from build123d import *

# Parameters (mm, degrees)
SKETCH1_R           = 17.5
BOSS_EXTRUDE1_DEPTH = 50
BOSS_EXTRUDE2_START = -50
SKETCH2_R           = 27.5
BOSS_EXTRUDE2_DEPTH = 10
FILLET1_R           = 3
SKETCH3_R           = 17
CUT_EXTRUDE1_DEPTH  = 50
SKETCH5_R           = 1.5
CUT_EXTRUDE4_DEPTH  = 10


with BuildPart() as part:
    # Sketch1 → Boss-Extrude1 (new body)
    with BuildSketch(Plane(origin=(0, 0, 0), x_dir=(1, 0, 0), z_dir=(0, 1, 0))):
        with Locations(Location((0, 0, 0), (0, 0, 90))):
            Circle(SKETCH1_R)
    extrude(amount=BOSS_EXTRUDE1_DEPTH)

    # Sketch2 → Boss-Extrude2 (add)
    with BuildSketch(Plane(origin=(0, 50, 0), x_dir=(1, 0, 0), z_dir=(0, 1, 0)).offset(BOSS_EXTRUDE2_START)):
        with Locations(Location((0, 0, 0), (0, 0, 270))):
            Circle(SKETCH2_R)
    extrude(amount=BOSS_EXTRUDE2_DEPTH)

    # Fillet1
    fillet1_edges = [part.edges().sort_by_distance(p)[0] for p in [
        (0, 50, 17.5),
        (0, 10, 17.5),
        (0, 10, -27.5),
    ]]
    fillet(fillet1_edges, radius=FILLET1_R)

    # Sketch3 → Cut-Extrude1 (cut)
    with BuildSketch(Plane(origin=(0, 50, 0), x_dir=(1, 0, 0), z_dir=(0, 1, 0))):
        with Locations(Location((0, 0, 0), (0, 0, 270))):
            Circle(SKETCH3_R)
    extrude(amount=-CUT_EXTRUDE1_DEPTH, mode=Mode.SUBTRACT)

    # Sketch5 → Cut-Extrude4 (cut)
    with BuildSketch(Plane(origin=(0, 10, 0), x_dir=(1, 0, 0), z_dir=(0, 1, 0))):
        with Locations(Location((-22.617014995, -0.042550907, 0), (0, 0, 270))):
            Circle(SKETCH5_R)
        with Locations(Location((-18.139935623, 13.821584384, 0), (0, 0, 270))):
            Circle(SKETCH5_R)
        with Locations(Location((-6.368768067, 22.406344218, 0), (0, 0, 270))):
            Circle(SKETCH5_R)
        with Locations(Location((8.200301755, 22.432642125, 0), (0, 0, 270))):
            Circle(SKETCH5_R)
        with Locations(Location((20.002384355, 13.890433198, 0), (0, 0, 270))):
            Circle(SKETCH5_R)
        with Locations(Location((24.529485319, 0.042550907, 0), (0, 0, 270))):
            Circle(SKETCH5_R)
        with Locations(Location((20.052405947, -13.821584384, 0), (0, 0, 270))):
            Circle(SKETCH5_R)
        with Locations(Location((8.28123839, -22.406344218, 0), (0, 0, 270))):
            Circle(SKETCH5_R)
        with Locations(Location((-6.287831432, -22.432642125, 0), (0, 0, 270))):
            Circle(SKETCH5_R)
        with Locations(Location((-18.089914032, -13.890433198, 0), (0, 0, 270))):
            Circle(SKETCH5_R)
    extrude(amount=-CUT_EXTRUDE4_DEPTH, mode=Mode.SUBTRACT)


solid = part.part
Part model, mm, in its own coordinate system. A direction names the side the tool comes from. Give positions to 0.01 mm unless a question says otherwise; leave off trailing zeros. Order: outer loops, then holes, each group sorted by start corner. A loop starts at its lowest first (then second) coordinate and runs counter-clockwise, first axis right, second up. Notation, with made-up numbers: (83, 44.25) -> (121, 44.25) arc R12 cw to (121, 62.25) -> close; hole circle Ø11 at (-11, -6.5). An arc over 180 degrees is marked (long way). Use one line per item in the form item = value.
(1) Saw through at A-A (x = 0). Write the cut outline in (y, z), then the cut area to 3 significant figures.
Solution:
outline = (0, -27.5) -> (7, -27.5) arc R3 ccw to (10, -24.5) -> (10, -20.5) arc R3 cw to (13, -17.5) -> (47, -17.5) arc R3 ccw to (48.66, -17) -> (0, -17) -> close; (0, 17) -> (48.66, 17) arc R3 ccw to (47, 17.5) -> (13, 17.5) arc R3 cw to (10, 20.5) -> (10, 24.5) arc R3 ccw to (7, 27.5) -> (0, 27.5) -> close
area = 248 mm²
(2) Saw through at D-D (y = 37.5). Write the cut outline in (x, z), then the cut area to 3 significant figures.
Solution:
outline = circle Ø35 at (0, 0); hole circle Ø34 at (0, 0)
area = 54.2 mm²
(3) Flat gauge pins, fed straight in: P1, Ø10, axis at y = 25.5, z = -19, coming from the +X side; P2, Ø4, axis at x = 20.05, z = 13.82, coming from the +Y side; P3, Ø10, axis at y = 29, z = -10, coming from the -X side. Where does each tip first touch, or does it go through?
Solution:
P1 = 10.5
P2 = 10
P3 = -16.77
(4) Saw through at C-C (y = 6). Count the separate pieces of the cut face and the enclosed holes in it, then the cut area to 3 significant figures.
Solution:
separate_pieces = 1
enclosed_holes = 11
area = 1,400 mm²
(5) Saw through at B-B (z = 0). Write the cut outline in (x, y), then the cut area to 3 significant figures.
Solution:
outline = (-27.5, 0) -> (-24.12, 0) -> (-24.12, 10) -> (-24.5, 10) arc R3 ccw to (-27.5, 7) -> close; (-21.12, 0) -> (-17, 0) -> (-17, 48.66) arc R3 ccw to (-17.5, 47) -> (-17.5, 13) arc R3 cw to (-20.5, 10) -> (-21.12, 10) -> close; (17, 0) -> (23.03, 0) -> (23.03, 10) -> (20.5, 10) arc R3 cw to (17.5, 13) -> (17.5, 47) arc R3 ccw to (17, 48.66) -> close; (26.03, 0) -> (27.5, 0) -> (27.5, 7) arc R3 ccw to (26.03, 9.58) -> close
area = 188 mm²
(6) Pull direction X, two halves, no side cores. Call faces 3 (the face through (21.016, 5.07, -14.996)), 4 (the face through (10.648, 29.762, 13.887)), 5 (the face through (0, 0, 18)): +X half, -X half, draft (parallel to the pull), parting line (faces both ways), or undercut.
Solution:
face_3 = undercut
face_4 = parting line
face_5 = draft
(7) Tool access for faces 1 (the face through (20, 10, 5.3)), 2 (the face through (-19.554, 5.07, 13.565)): list every direction of +Z, -Z, +X, -X, +Y, -Y with a clear straight run to the whole face (end or side of a thin tool).
Solution:
face_1 = +Y
face_2 = +Y, -Y
(8) Drill centre lines: line 1 (X direction, y = 8, z = -1); line 2 (X direction, y = 7.5, z = 21.5); line 3 (Z direction, x = -12, y = 9.5). Where is each one in solid material? Low to high. Write a range as from..to.
Solution:
line_1 = -27.31..-23.7, -21.54..-16.97, 16.97..23.37, 25.68..27.31
line_2 = -17.08..-7.46, -5.11..7.09, 9.48..17.08
line_3 = -23.24..-12.04, 12.04..23.24
